Input: dimensioned drawing with shaded views. Units: mm. Origin: part minimum x, y, z. Give positions to 0.01 mm unless a question says otherwise; leave off trailing zeros. Loops run counter-clockwise (first coordinate to the right, second up) from the corner with the lowest first, then second, coordinate; pieces in that order, holes last.
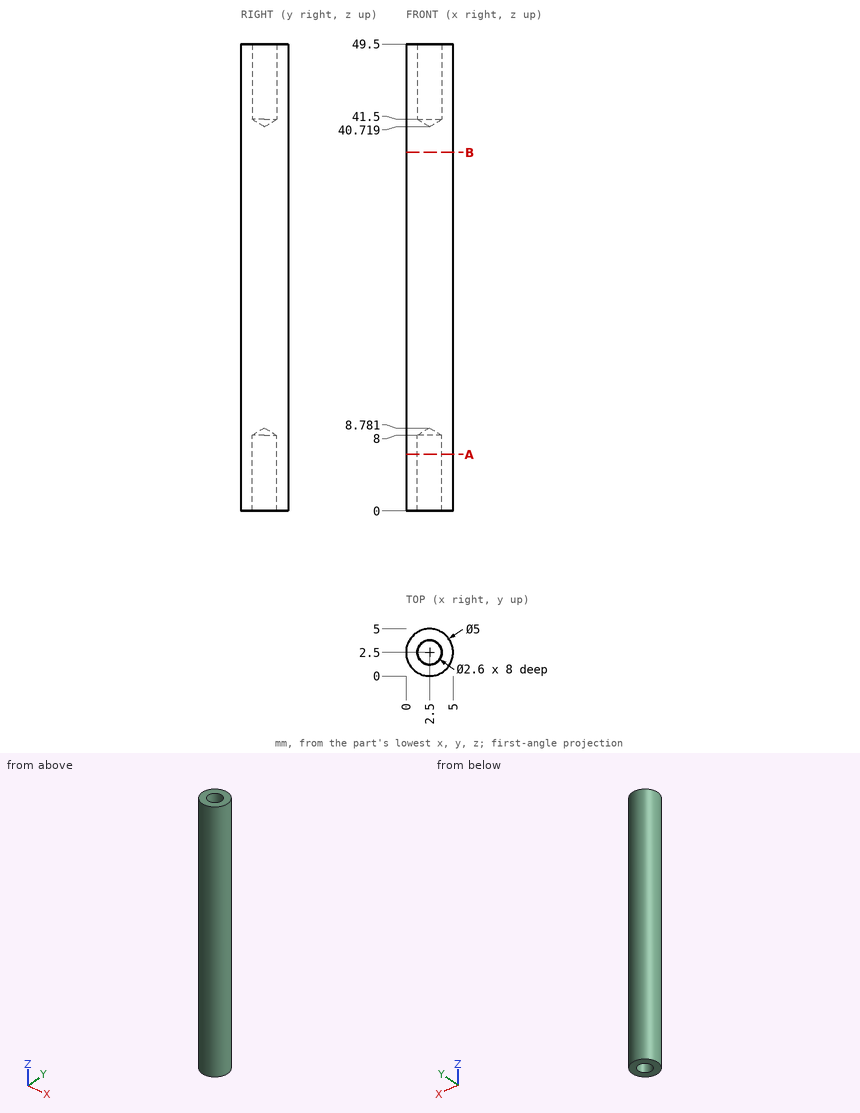
Item 1: Ray query, probe 1 along Y at (x, z) = (2.5, 45.5); probe 2 along X at (y, z) = (3.6, 4) (1 decimal); probe 3 along X at (y, z) = (3.1, 47). Return the intervals inside material, ascending.
Values follow:
probe 1: y = 0 to 1.2, 3.8 to 5
probe 2: x = 0.3 to 1.8, 3.2 to 4.7
probe 3: x = 0.07 to 1.35, 3.65 to 4.93
Item 2: Section query A-A on z = 6. Return loops of the section in (x, y), plus the area to 3 significant figures.
Values follow:
outline: circle Ø5 at (2.5, 2.5); hole circle Ø2.6 at (2.5, 2.5)
area: 14.3 mm2
Item 3: Section query B-B on z = 38. Return loops of the section in (x, y).
Values follow:
outline: circle Ø5 at (2.5, 2.5)
Item 4: Pin query (flat end, axial travel): pin 1 (1 mm diameter, centred on y = 3.5, z = 9, fed in from +X); pin 2 (1.6 mm diameter, centred on x = 2.5, y = 2.5, fed in from +Z); pin 3 (2.5 mm diameter, centred on x = 2.5, y = 2.5, fed in from +Z). Return the tip coordinate at first contact, or that it passes through.
Values follow:
pin 1: stops at x = 4.95
pin 2: stops at z = 41.2
pin 3: stops at z = 41.47
